```python
from build123d import *

# Parameters (mm, degrees)
SKETCH1_R          = 3.025
BASE_FLANGE1_DEPTH = 1


# Sheet-metal steps are written as plain solids
with BuildPart() as part:
    # Sketch1 → Base-Flange1 (new body)
    with BuildSketch(Plane.XY):
        with BuildLine():
            Line((6.5, 0), (6.5, 3.105048502))
            ThreePointArc((6.5, 3.105048502), (6.430087021, 3.472387764), (6.230123733, 3.788363462))
            Line((6.230123733, 3.788363462), (4.019876267, 6.150018373))
            ThreePointArc((4.019876267, 6.150018373), (3.819912979, 6.465994071), (3.75, 6.833333333))
            Line((3.75, 6.833333333), (3.75, 16))
            ThreePointArc((3.75, 16), (3.457106781, 16.707106781), (2.75, 17))
            Line((2.75, 17), (-2.75, 17))
            ThreePointArc((-2.75, 17), (-3.457106781, 16.707106781), (-3.75, 16))
            Line((-3.75, 16), (-3.75, 6.833333333))
            ThreePointArc((-3.75, 6.833333333), (-3.819912979, 6.465994071), (-4.019876267, 6.150018373))
            Line((-4.019876267, 6.150018373), (-6.230123733, 3.788363462))
            ThreePointArc((-6.230123733, 3.788363462), (-6.430087021, 3.472387764), (-6.5, 3.105048502))
            Line((-6.5, 3.105048502), (-6.5, 0))
            ThreePointArc((-6.5, 0), (0, -6.5), (6.5, 0))
        make_face()
        Circle(SKETCH1_R, mode=Mode.SUBTRACT)
    extrude(amount=-BASE_FLANGE1_DEPTH)


solid = part.part
```
The listing builds one solid part. Answer for the finished solid, in the listing's coordinates (mm). A direction names the side the tool comes from. Coordinates: 2 decimals unless noted, no trailing zeros. Loops run counter-clockwise (first coordinate to the right, second up) from the corner with the lowest first, then second, coordinate; pieces in that order, holes last. Notation, with made-up numbers: M -16,39.5 L -6,39.5 A28 ccw -6,77.5 Z; hole C 39.5,-10 d3. An arc over 180 degrees is marked long. Answer as a JSON object with one key per item and string values. Group by question number.
Item 1: Section D-D (y = 8.5) is taken. Write down the section's boundary in (x, z), and give its area (3 significant figures).
Item 2: Section A-A (x = 0) is taken. Write down the section's boundary in (y, z) (3 decimals).
Item 3: Section B-B (z = -0.7) is taken. Write down the section's boundary in (x, y) (3 decimals), and give its area (3 significant figures).
Item 4: Determine the mould class of faces 4 (the face through (-6.5, 1.6, -0.5)), 5 (the face through (-3.449, 16.715, -0.493)), 6 (the face through (2.794, -1.159, -0.493)), 7 (the face through (-0.1, -6.5, -0.5)) for opening direction Y: +Y half, -Y half, draft (parallel to the pull), parting line (faces both ways), or undercut.
Item 5: Section C-C (y = 0.5) is taken. Write down the section's boundary in (x, z), and give its area (3 significant figures).
Item 6: Consider L1, parallel to Y at x = 0, z = -0.65 (3 decimals); L2, parallel to Y at x = 2, z = -0.5; L3, parallel to X at y = -0.75, z = -0.9. Determine where each line is inside the solid, lowest interval first.
Item 7: Which of the six approach directions +Z, -Z, +X, -X, +Y, -Y give full straight-line access (tool end or side, diameter ignored) to faces 1 (the face through (0, 5, 0)), 2 (the face through (3.75, 11.4, -0.5)), 3 (the face through (-3.75, 11.5, -0.5))?
Solved:
{
 "1": {"outline": "M -3.75,-1 L 3.75,-1 L 3.75,0 L -3.75,0 Z", "area": "7.50 mm2"},
 "2": {"outline": "M -6.5,-1 L -3.025,-1 L -3.025,0 L -6.5,0 Z; M 3.025,-1 L 17,-1 L 17,0 L 3.025,0 Z"},
 "3": {"outline": "M -6.5,0 A6.5 ccw 6.5,0 L 6.5,3.105 A1 ccw 6.23,3.788 L 4.02,6.15 A1 cw 3.75,6.833 L 3.75,16 A1 ccw 2.75,17 L -2.75,17 A1 ccw -3.75,16 L -3.75,6.833 A1 cw -4.02,6.15 L -6.23,3.788 A1 ccw -6.5,3.105 Z; hole C 0,0 d6.05", "area": "192 mm2"},
 "4": {"face 4": "draft", "face 5": "+Y half", "face 6": "undercut", "face 7": "-Y half"},
 "5": {"outline": "M -6.5,-1 L -2.98,-1 L -2.98,0 L -6.5,0 Z; M 2.98,-1 L 6.5,-1 L 6.5,0 L 2.98,0 Z", "area": "7.03 mm2"},
 "6": {"L1": "y = -6.5 to -3.025, 3.025 to 17", "L2": "y = -6.18 to -2.27, 2.27 to 17", "L3": "x = -6.46 to -2.93, 2.93 to 6.46"},
 "7": {"face 1": "+Z, +X, -X, +Y, -Y", "face 2": "+Z, -Z, +X, +Y", "face 3": "+Z, -Z, -X, +Y"}
}
